Source: CAD feature listing. Evaluate the final solid. Frame: model axes, mm. Face numbers are marked on the shaded views. A direction names the side the tool comes from. Coordinates: 2 decimals unless noted, no trailing zeros. Order: outer loops, then holes, each group sorted by start corner. A loop starts at its lowest first (then second) coordinate and runs counter-clockwise, first axis right, second up.
Item 1: Mould query, pull axis X, two halves, no side actions, for the marked faces 1, 2 and 3. Classes: released by +X, released by -X, zero draft, split by the parting line, or undercut.
Item 2: Ray query, line 1 (Y direction, x = -15, z = 13); line 2 (Y direction, x = -15, z = 19) (3 decimals); line 3 (Z direction, x = 15, y = -13). Return the intervals inside material, ascending.
Item 3: Section C-C on z = 4. Return the cut outline in (x, y).
Item 4: Section D-D on z = 14. Return the cut outline in (x, y).
Item 5: Section B-B on x = 0. Return the cut outline in (y, z).
Item 6: Contact query for flat-ended pins moving along their axis: P1, Ø3.5, axis at x = 0, y = 3, coming from the -Z side; P2, Ø3, axis at y = -11.5, z = 12.5, coming from the +X side; P3, Ø3.5, axis at x = -0.5, z = -6.5, coming from the -Y side; P4, Ø8, axis at x = 12.5, z = -4.5, coming from the +Y side. Output: stop coordinate, or through.
Item 7: Section A-A on z = -7. Return the cut outline in (x, y), then the cut area to 3 significant figures.
Item 8: Reachability of the marked faces 4, 5 and 6 from +Z, -Z, +X, -X, +Y, -Y: full face, straight path, thin tool, end or side. Return the list, or none.
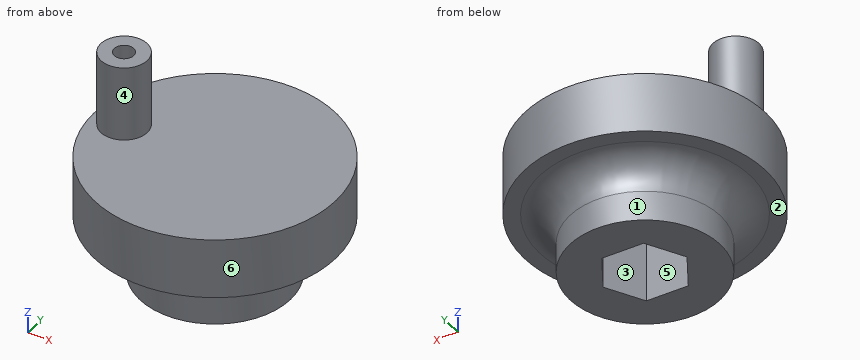
from build123d import *

# Parameters (mm, degrees)
SKETCH1_R           = 20
BOSS_EXTRUDE1_DEPTH = 10
SKETCH2_R           = 3.85
BOSS_EXTRUDE2_DEPTH = 12.5
SKETCH3_R           = 12.5
BOSS_EXTRUDE3_DEPTH = 10
SKETCH5_R           = 1.5
CUT_EXTRUDE1_DEPTH  = 16.5
SKETCH6_R           = 1.625
CUT_EXTRUDE2_DEPTH  = 5.2
FILLET1_R           = 5


with BuildPart() as part:
    # Sketch1 → Boss-Extrude1 (new body)
    with BuildSketch(Plane.XY):
        Circle(SKETCH1_R)
    extrude(amount=BOSS_EXTRUDE1_DEPTH)

    # Sketch2 → Boss-Extrude2 (add)
    with BuildSketch(Plane.XY.offset(10)):
        with Locations((-15, 0)):
            Circle(SKETCH2_R)
    extrude(amount=BOSS_EXTRUDE2_DEPTH)

    # Sketch3 → Boss-Extrude3 (add)
    with BuildSketch(Plane(origin=(0, 0, 0), x_dir=(-1, 0, 0), z_dir=(0, 0, -1))):
        with Locations(Location((0, 0, 0), (0, 0, 180))):
            Circle(SKETCH3_R)
        Polygon((3.464101615, 6), (-3.464101615, 6), (-6.92820323, 0), (-3.464101615, -6), (3.464101615, -6), (6.92820323, 0), align=None, mode=Mode.SUBTRACT)
    extrude(amount=BOSS_EXTRUDE3_DEPTH)

    # Sketch5 → Cut-Extrude1 (cut)
    with BuildSketch(Plane.XY.offset(22.5)):
        with Locations((-15, 0)):
            Circle(SKETCH5_R)
    extrude(amount=-CUT_EXTRUDE1_DEPTH, mode=Mode.SUBTRACT)

    # Sketch6 → Cut-Extrude2 (cut)
    with BuildSketch(Plane.XY.offset(22.5)):
        with Locations((-15, 0)):
            Circle(SKETCH6_R)
    extrude(amount=-CUT_EXTRUDE2_DEPTH, mode=Mode.SUBTRACT)

    # Fillet1
    fillet1_edges = [part.edges().sort_by_distance(p)[0] for p in [
        (-12.5, 0, 0),
    ]]
    fillet(fillet1_edges, radius=FILLET1_R)


solid = part.part
Answer list:
1. face 1: split by the parting line
1. face 2: zero draft
1. face 3: undercut
2. line 1: y = -3.85 to -1.5, 1.5 to 3.85
2. line 2: y = -3.85 to -1.625, 1.625 to 3.85
2. line 3: z = 0 to 10
3. outline: circle Ø40 at (0, 0)
4. outline: circle Ø7.7 at (-15, 0); hole circle Ø3 at (-15, 0)
5. outline: (-20, 0) - (-17.5, 0) arc R5 cw to (-12.5, -5) - (-12.5, -10) - (-6, -10) - (-6, 0) - (6, 0) - (6, -10) - (12.5, -10) - (12.5, -5) arc R5 cw to (17.5, 0) - (20, 0) - (20, 10) - (-20, 10) - close
6. P1: stops at z = 0
6. P2: passes through
6. P3: stops at y = -12.5
6. P4: stops at y = 9.93
7. outline: circle Ø25 at (0, 0); hole (-6.93, 0) - (-3.46, -6) - (3.46, -6) - (6.93, 0) - (3.46, 6) - (-3.46, 6) - close
7. area: 366 mm2
8. face 4: +Z
8. face 5: -Z
8. face 6: +Z, -Z
